from build123d import *

# Parameters (mm, degrees)
SKETCH_2_R      = 16
EXTRUDE_5_DEPTH = 15
SKETCH_2_11_R   = 55
SKETCH_2_11_R_2 = 45
EXTRUDE_6_DEPTH = 11
SKETCH_2_20_R   = 45
SKETCH_2_20_R_2 = 12
SKETCH_2_20_R_3 = 16
EXTRUDE_9_DEPTH = 3


# Read off the part's stored shape, not the designer's step: the other step
with BuildPart() as part:
    # Sketch 2 → Extrude 5 (new, symmetric)
    with BuildSketch(Plane.XY):
        Circle(SKETCH_2_R)
        with BuildLine():
            ThreePointArc((-3.410963595, 6.679470589), (0, -7.5), (3.410963595, 6.679470589))
            Line((3.410963595, 6.679470589), (3.410963595, 9.309886023))
            Line((3.410963595, 9.309886023), (-3.410963595, 9.309886023))
            Line((-3.410963595, 9.309886023), (-3.410963595, 6.679470589))
        make_face(mode=Mode.SUBTRACT)
    extrude(amount=EXTRUDE_5_DEPTH, both=True)



with BuildPart() as body_2:
    # Sketch 2_11 → Extrude 6 (new, symmetric)
    with BuildSketch(Plane.XY):
        Circle(SKETCH_2_11_R)
        Circle(SKETCH_2_11_R_2, mode=Mode.SUBTRACT)
    extrude(amount=EXTRUDE_6_DEPTH, both=True)

    # Other 6 outline → Other 6 (revolve, cut)
    with BuildSketch(Plane.XZ):
        Polygon((55, -2), (50, -3.721638066), (50, -6.721638066), (55, -8.443276133), align=None)
        Polygon((50, 3.721638066), (55, 2), (55, 8.443276133), (50, 6.721638066), align=None)
    revolve(axis=Axis((0, 0, 0), (0, 0, 1)), mode=Mode.SUBTRACT)


with BuildPart() as part_1:
    add(part.part)

    add(body_2.part)  # Extrude 9 merges body 2
    # Sketch 2_20 → Extrude 9 (add, symmetric)
    with BuildSketch(Plane.XY):
        Circle(SKETCH_2_20_R)
        with Locations((-29.998597199, -0.290113977)):
            Circle(SKETCH_2_20_R_2, mode=Mode.SUBTRACT)
        with Locations((-15.250544673, 25.834490264)):
            Circle(SKETCH_2_20_R_2, mode=Mode.SUBTRACT)
        with Locations((14.748052526, 26.12460424)):
            Circle(SKETCH_2_20_R_2, mode=Mode.SUBTRACT)
        with Locations((29.998597199, 0.290113977)):
            Circle(SKETCH_2_20_R_2, mode=Mode.SUBTRACT)
        with Locations((15.250544673, -25.834490264)):
            Circle(SKETCH_2_20_R_2, mode=Mode.SUBTRACT)
        with Locations((-14.748052526, -26.12460424)):
            Circle(SKETCH_2_20_R_2, mode=Mode.SUBTRACT)
        Circle(SKETCH_2_20_R_3, mode=Mode.SUBTRACT)
    extrude(amount=EXTRUDE_9_DEPTH, both=True)


solid = part_1.part
CAD build for the part. Positions are in the model's coordinates, mm. A direction names the side the tool comes from. Coordinates: 2 decimals unless noted, no trailing zeros. Loops run counter-clockwise (first coordinate to the right, second up) from the corner with the lowest first, then second, coordinate; pieces in that order, holes last. Notation, with made-up numbers: (1, -20) - (22, -20) arc R33 ccw to (22, 18) - close; hole circle Ø7 at (-30, 69). An arc over 180 degrees is marked (long way). Use one line per item in the form item = value. Start each with the question number.
1) Tool access for faces 4 (the face through (-3.47, -15.62, -8.92)), 5 (the face through (0, 9.31, 0)), 6 (the face through (20.765, -39.923, 6.944)), 7 (the face through (47.69, 15.02, 5.2)): list every direction of +Z, -Z, +X, -X, +Y, -Y with a clear straight run to the whole face (end or side of a thin tool).
2) Drill centre lines: L1, parallel to Y at x = 0, z = -6; L2, parallel to Y at x = 0, z = -0.25; L3, parallel to Z at x = -48.5, y = 25. Where is each one in solid material? Low to high. Write a range as from..to.
3) Band-saw the part on A-A (z = 5). Give the cut face in (x, y).
4) Band-saw the part on B-B (x = -20.5). State how many separate pieces and enclosed holes the cut face has, and give its area (3 significant figures).
5) Flat gauge pins, fed straight in: pin 1 (1.5 mm diameter, centred on x = -0.5, y = 33, fed in from +Z); pin 2 (7.5 mm diameter, centred on x = 1.5, z = 3, fed in from -Y); pin 3 (1 mm diameter, centred on y = -1, z = 10.5, fed in from +X); pin 4 (14.5 mm diameter, centred on x = 30, y = 0.29, fed in from +Z). Where does each tip first touch, or does it go through?
6) Two-plate mould, pull along Y, no slides. Class faces 1 (the face through (-11.923, -53.692, -9.704)), 2 (the face through (3.33, -6.89, 15)), 3 (the face through (26.696, -22.23, -0.042)): +Y half, -Y half, draft (parallel to the pull), parting line (faces both ways), or undercut.
Check values:
q1.face_4 = -Z
q1.face_5 = +Z, -Z
q1.face_6 = +Z
q1.face_7 = none
q2.L1 = -50..-45, -16..-7.5, 9.31..16, 45..50
q2.L2 = -55..-7.5, 9.31..55
q2.L3 = -11..-8.29, -2.15..2.15, 8.29..11
q3.outline = circle Ø100 at (0, 0); circle Ø32 at (0, 0); hole circle Ø90 at (0, 0); hole (-3.41, 6.68) arc R7.5 ccw (long way) to (3.41, 6.68) - (3.41, 9.31) - (-3.41, 9.31) - close
q4.separate_pieces = 4
q4.enclosed_holes = 0
q4.area = 517 mm2
q5.pin_1 = 3
q5.pin_2 = -55
q5.pin_3 = 55
q5.pin_4 = through
q6.face_1 = parting line
q6.face_2 = draft
q6.face_3 = undercut
